Check sheet for the modelled part. Datum: model origin and axes. Units: mm. A direction names the side the tool comes from. Give positions to 0.01 mm unless a question says otherwise; leave off trailing zeros. Write each loop counter-clockwise with the first axis right and the second up, starting at its lowest first coordinate (ties: lowest second). Pieces come first, ordered by that corner, then holes.
from build123d import *

# Parameters (mm, degrees)
SKETCH1_R           = 250
BOSS_EXTRUDE1_DEPTH = 2200
SHELL1_T            = -2
SKETCH10_R          = 250
SKETCH10_R_2        = 100
BOSS_EXTRUDE4_DEPTH = 2
SKETCH11_R          = 102
SKETCH11_R_2        = 100
EXTRUDE_THIN2_DEPTH = 150


with BuildPart() as part:
    # Sketch1 → Boss-Extrude1 (new body)
    with BuildSketch(Plane.XY):
        Circle(SKETCH1_R)
    extrude(amount=BOSS_EXTRUDE1_DEPTH)

    # Shell1
    shell1_openings = [part.faces().sort_by_distance(p)[0] for p in [
        (0, 0, 2200),
    ]]
    offset(amount=SHELL1_T, openings=shell1_openings, kind=Kind.INTERSECTION)

    # Sketch10 → Boss-Extrude4 (add)
    with BuildSketch(Plane.XY.offset(2200)):
        Circle(SKETCH10_R)
        Circle(SKETCH10_R_2, mode=Mode.SUBTRACT)
    extrude(amount=BOSS_EXTRUDE4_DEPTH)

    # Sketch11 → Extrude-Thin2 (add)
    with BuildSketch(Plane.XY.offset(2202)):
        Circle(SKETCH11_R)
        Circle(SKETCH11_R_2, mode=Mode.SUBTRACT)
    extrude(amount=EXTRUDE_THIN2_DEPTH)


solid = part.part
1) Scan lines: L1, parallel to Y at x = 0, z = 2233.5; L2, parallel to Z at x = 158, y = -45.5; L3, parallel to Y at x = 0, z = 1486. Record each from-to range of solid material in increasing order.
2) Sectioned sample at C-C on z = 1035. Record the boundary of the cut face in (x, y), then the cut area to 3 significant figures.
3) Gauge pin test, flat ends, axial feed: pin 1 (4 mm diameter, centred on x = 136, z = 1205.5, fed in from +Y); pin 2 (12 mm diameter, centred on y = -114.5, z = 1169, fed in from -X); pin 3 (2 mm diameter, centred on x = 39.5, y = -99.5, fed in from +Z). Record the tip position at first contact, or that the pin passes through.
4) Sectioned sample at A-A on x = 166.5. Record the boundary of the cut face in (y, z).
5) Access from +Z, -Z, +X, -X, +Y, -Y to the whole of each face (thin tool, end or side, straight path). Record for faces 1 (the cylindrical face through (-22.112, -99.574, 2275.95)), 2 (the flat face through (-3, 4, 0)), 3 (the flat face through (-3, -107, 2200)).
6) Sectioned sample at D-D on y = 0. Record the boundary of the cut face in (x, z), then the cut area to 3 significant figures.
7) Draft check along X on faces 4 (the cylindrical face through (-249.76, 10.99, 1085.59)), 5 (the flat face through (-3, -108, 2202)), 6 (the cylindrical face through (95.38, 30.04, 2274.94)). Enter one of: +X half, -X half, draft (parallel to the pull), parting line (faces both ways), or undercut.
8) Sectioned sample at B-B on y = 156.5. Record the boundary of the cut face in (x, z).
Answers below:
1. L1: y = -102 to -100, 100 to 102
1. L2: z = 0 to 2, 2200 to 2202
1. L3: y = -250 to -248, 248 to 250
2. outline: circle Ø500 at (0, 0); hole circle Ø496 at (0, 0)
2. area: 3,130 mm2
3. pin 1: stops at y = 211.05
3. pin 2: stops at x = -225.23
3. pin 3: stops at z = 2202
4. outline: (-186.49, 0) - (186.49, 0) - (186.49, 2202) - (-186.49, 2202) - close; hole (-183.8, 2) - (183.8, 2) - (183.8, 2200) - (-183.8, 2200) - close
5. face 1: +Z
5. face 2: -Z, +X, -X, +Y, -Y
5. face 3: none
6. outline: (-250, 0) - (250, 0) - (250, 2202) - (102, 2202) - (102, 2352) - (100, 2352) - (100, 2200) - (248, 2200) - (248, 2) - (-248, 2) - (-248, 2200) - (-100, 2200) - (-100, 2352) - (-102, 2352) - (-102, 2202) - (-250, 2202) - close
6. area: 11,000 mm2
7. face 4: parting line
7. face 5: draft
7. face 6: undercut
8. outline: (-194.96, 0) - (194.96, 0) - (194.96, 2202) - (-194.96, 2202) - close; hole (-192.38, 2) - (192.38, 2) - (192.38, 2200) - (-192.38, 2200) - close
